```python
from build123d import *

# Parameters (mm, degrees)
SKETCH1_W            = 60
SKETCH1_H            = 7.5
BOSS_EXTRUDE1_DEPTH  = 13
SKETCH3_W            = 12
SKETCH3_H            = 5
CUT_EXTRUDE1_DEPTH   = 10.5
SKETCH4_R            = 1
CUT_EXTRUDE2_DEPTH   = 10
SKETCH9_W            = 45.277568689
SKETCH9_H            = 2.15
CUT_EXTRUDE8_DEPTH   = 15
SKETCH13_W           = 45.277568689
SKETCH13_H           = 3.2
CUT_EXTRUDE10_DEPTH  = 8
SKETCH14_W           = 45.277568689
SKETCH14_H           = 0.95
CUT_EXTRUDE11_DEPTH  = 2.2
RIB10_REACH          = 34.91
SKETCH16_WALL_W      = 80.220727034
SKETCH16_WALL_H      = 1.3
SKETCH20_W           = 12
SKETCH20_H           = 5
BOSS_EXTRUDE3_DEPTH  = 3
SKETCH22_W           = 12
SKETCH22_H           = 5
CUT_EXTRUDE13_DEPTH  = 1.95
CUT_EXTRUDE14_START  = -10
SKETCH23_R           = 1
CUT_EXTRUDE14_DEPTH  = 10
SCALE1_SCALE         = 1.6
SCALE3_SCALE         = 0.8
SCALE4_SCALE         = 0.95890411
SKETCH34_W           = 14.546034326
SKETCH34_H           = 7.999999695
CUT_EXTRUDE20_DEPTH  = 15
SKETCH39_W           = 3.927671232
SKETCH39_H           = 3.436712329
BOSS_EXTRUDE5_DEPTH  = 25
BOSS_EXTRUDE6_DEPTH  = 2
FILLET1_R            = 15
FILLET3_R            = 5
BOSS_EXTRUDE7_DEPTH  = 2
FILLET4_R            = 5
FILLET5_R            = 5
FILLET6_R            = 5
FILLET7_R            = 5
SKETCH52_W           = 9.205479452
SKETCH52_H           = 15.956164384
CUT_EXTRUDE21_DEPTH  = 0.05
SKETCH54_W           = 0.182732797
SKETCH54_H           = 6.136986302
BOSS_EXTRUDE8_DEPTH  = 15
SKETCH55_W           = 6.136986302
SKETCH55_H           = 3.40109589
CUT_EXTRUDE22_DEPTH  = 15
SKETCH57_W           = 14.496034326
SKETCH57_H           = 7.999999695
CUT_EXTRUDE23_DEPTH  = 12.16
SKETCH58_W           = 18.020271855
SKETCH58_H           = 15.956164384
BOSS_EXTRUDE9_DEPTH  = 3
SKETCH59_W           = 18.020271855
SKETCH59_H           = 15.956164384
BOSS_EXTRUDE10_DEPTH = 3


with BuildPart() as part:
    # Sketch1 → Boss-Extrude1 (new body)
    with BuildSketch(Plane(origin=(0, 0, 0), x_dir=(1, 0, 0), z_dir=(0, 1, 0))):
        Rectangle(SKETCH1_W, SKETCH1_H)
    extrude(amount=BOSS_EXTRUDE1_DEPTH)

    # Sketch3 → Cut-Extrude1 (cut)
    with BuildSketch(Plane(origin=(0, 13, 0), x_dir=(1, 0, 0), z_dir=(0, 1, 0))):
        with Locations((-24, 0)):
            Rectangle(SKETCH3_W, SKETCH3_H)
    extrude(amount=-CUT_EXTRUDE1_DEPTH, mode=Mode.SUBTRACT)

    # Sketch4 → Cut-Extrude2 (cut)
    with BuildSketch(Plane(origin=(0, 2.5, 0), x_dir=(1, 0, 0), z_dir=(0, 1, 0))):
        with Locations(Location((-21, 0, 0), (0, 0, 270))):
            Circle(SKETCH4_R)
        with Locations(Location((-26.7, 0, 0), (0, 0, 270))):
            Circle(SKETCH4_R)
    extrude(amount=-CUT_EXTRUDE2_DEPTH, mode=Mode.SUBTRACT)

    # Sketch9 → Cut-Extrude8 (cut)
    with BuildSketch(Plane.XZ):
        with Locations((7.361215656, 2.675)):
            Rectangle(SKETCH9_W, SKETCH9_H)
        with Locations((7.361215656, -2.675)):
            Rectangle(SKETCH9_W, SKETCH9_H)
    extrude(amount=-CUT_EXTRUDE8_DEPTH, mode=Mode.SUBTRACT)

    # Sketch13 → Cut-Extrude10 (cut)
    with BuildSketch(Plane.XZ):
        with Locations((7.361215656, 0)):
            Rectangle(SKETCH13_W, SKETCH13_H)
    extrude(amount=-CUT_EXTRUDE10_DEPTH, mode=Mode.SUBTRACT)

    # Sketch14 → Cut-Extrude11 (cut)
    with BuildSketch(Plane.XZ.offset(-8)):
        with Locations((7.361215656, 1.125)):
            Rectangle(SKETCH14_W, SKETCH14_H)
        with Locations((7.361215656, -1.125)):
            Rectangle(SKETCH14_W, SKETCH14_H)
    extrude(amount=-CUT_EXTRUDE11_DEPTH, mode=Mode.SUBTRACT)

    # Sketch16 wall → Rib10 (add, up to next)
    with BuildSketch(Plane(origin=(-10.539893857, 4, 0), x_dir=(-0.764085816902, -0.645114613389, 0), z_dir=(0.645114613389, -0.764085816902, 0)), mode=Mode.PRIVATE) as rib10_sk1:
        Rectangle(SKETCH16_WALL_W, SKETCH16_WALL_H)
    rib10_tool1 = extrude(rib10_sk1.sketch, amount=-RIB10_REACH, mode=Mode.PRIVATE) - part.part
    add(rib10_tool1.solids().sort_by_distance((-10.539893857, 4, 0))[0])

    # Sketch20 → Boss-Extrude3 (add)
    with BuildSketch(Plane(origin=(0, 2.5, 0), x_dir=(1, 0, 0), z_dir=(0, 1, 0))):
        with Locations((-24, 0)):
            Rectangle(SKETCH20_W, SKETCH20_H)
    extrude(amount=BOSS_EXTRUDE3_DEPTH)

    # Sketch22 → Cut-Extrude13 (cut)
    with BuildSketch(Plane(origin=(0, 5.5, 0), x_dir=(1, 0, 0), z_dir=(0, 1, 0))):
        with Locations((-24, 0)):
            Rectangle(SKETCH22_W, SKETCH22_H)
    extrude(amount=-CUT_EXTRUDE13_DEPTH, mode=Mode.SUBTRACT)

    # Sketch23 → Cut-Extrude14 (cut)
    with BuildSketch(Plane.XZ.offset(CUT_EXTRUDE14_START)):
        with Locations(Location((-26.7, 0, 0), (0, 0, 90))):
            Circle(SKETCH23_R)
        with Locations(Location((-21, 0, 0), (0, 0, 90))):
            Circle(SKETCH23_R)
    extrude(amount=CUT_EXTRUDE14_DEPTH, mode=Mode.SUBTRACT)


with BuildPart() as part_1:
    # Scale1: scaled about (-10.495093685, 7.511594664, 0)
    add(part.part.scale(SCALE1_SCALE).moved(Location((6.297056211, -4.506956798, 0))))


with BuildPart() as part_2:
    # Scale3: scaled about (-10.495093686, 7.511594664, 0)
    add(part_1.part.scale(SCALE3_SCALE).moved(Location((-2.099018737, 1.502318933, 0))))


with BuildPart() as part_3:
    # Scale4: scaled about (-10.495093686, 7.511594664, 0)
    add(part_2.part.scale(SCALE4_SCALE).moved(Location((-0.43130522, 0.308695671, 0))))

    # Sketch34 → Cut-Extrude20 (cut)
    with BuildSketch(Plane(origin=(0, 2.649144227, 0), x_dir=(1, 0, 0), z_dir=(0, 1, 0))):
        with Locations((-27.162345095, -7.59e-07)):
            Rectangle(SKETCH34_W, SKETCH34_H)
    extrude(amount=CUT_EXTRUDE20_DEPTH, mode=Mode.SUBTRACT)

    # Sketch39 → Boss-Extrude5 (add)
    with BuildSketch(Plane(origin=(39.208473359, 0, 0), x_dir=(0, 0, -1), z_dir=(1, 0, 0))):
        with Locations((0, 12.529692173)):
            Rectangle(SKETCH39_W, SKETCH39_H)
    extrude(amount=BOSS_EXTRUDE5_DEPTH)

    # Sketch45 → Boss-Extrude6 (add)
    with BuildSketch(Plane.XY.offset(1.963835616)):
        Polygon((64.208473359, 14.248048337), (67.197905162, 11.258616533), (67.903164447, 7.966965022), (68.244364149, 4.408739558), (65.703189261, 8.649364426), (64.208473359, 10.811336008), align=None)
    extrude(amount=-BOSS_EXTRUDE6_DEPTH)

    # Fillet1
    # the kernel refuses this fillet: 15 mm, written as the material it takes off along each edge
    with BuildSketch(Plane(origin=(67.197905162, 11.258616533, 12.842753048), x_dir=(-0.7071067811865568, 0.7071067811865384, 0), z_dir=(0, 0, -1))) as fillet1_piece_1:
        with BuildLine():
            CenterArc((4.351566973, -15), FILLET1_R, 90, 28.588827617)
            Line((-2.826242727, -1.828855482), (0, 0))
            Line((0, 0), (4.351566973, 0))
        make_face()
    extrude(amount=23.757834864, mode=Mode.SUBTRACT)

    # Fillet3
    fillet3_edges = [part_3.edges().sort_by_distance(p)[0] for p in [
        (64.207755923, 14.248048337, 0),
    ]]
    fillet(fillet3_edges, radius=FILLET3_R)

    # Sketch47 → Boss-Extrude7 (add)
    with BuildSketch(Plane.XY.offset(1.963835616)):
        Polygon((62.681686065, 10.811336008), (65.137458222, 8.07903323), (66.974128155, 4.550150551), (68.244364149, 4.408739558), (65.703189261, 8.649364426), (64.208473359, 10.811336008), align=None)
    extrude(amount=-BOSS_EXTRUDE7_DEPTH)

    # Fillet4
    fillet4_edges = [part_3.edges().sort_by_distance(p)[0] for p in [
        (62.681686065, 10.811336008, 0.963835616),
    ]]
    fillet(fillet4_edges, radius=FILLET4_R)

    # Fillet5
    fillet5_edges = [part_3.edges().sort_by_distance(p)[0] for p in [
        (65.137458222, 8.07903323, 0.963835616),
    ]]
    fillet(fillet5_edges, radius=FILLET5_R)

    # Fillet6
    # the kernel refuses this fillet: 5 mm, written as the material it takes off along each edge
    with BuildSketch(Plane(origin=(68.244364149, 4.408739558, 10.889498263), x_dir=(-0.993860211442073, 0.11064303011178676, 0), z_dir=(0, 0, -1))) as fillet6_piece_1:
        with BuildLine():
            CenterArc((5.625725169, 2.469414691), FILLET6_R, 168.170246518, 41.425870444)
            Line((0.731919855, 3.494436423), (0.634043748, 3.514936858))
            Line((0.634043748, 3.514936858), (-0.097876106, 0.020500435))
            Line((-0.097876106, 0.020500435), (0, -0.1))
            ThreePointArc((0, -0.1), (0.639041577, -0.1), (1.191130314, -0.049388294))
            Line((1.191130314, -0.049388294), (1.278083154, 0))
        make_face()
    extrude(amount=19.851325293, mode=Mode.SUBTRACT)

    # Fillet7
    # the kernel refuses this fillet: 5 mm, written as the material it takes off along each edge
    with BuildSketch(Plane(origin=(39.208473358, 8.111062035, -11.897149471), x_dir=(1.1344900488242768e-10, 1.0, 0), z_dir=(0, 0, 1))) as fillet7_piece_1:
        with BuildLine():
            CenterArc((4.999999999, 4.439736501), FILLET7_R, 180.000000007, 62.61642823)
            Line((-1e-09, 4.439736501), (-0.100000001, 4.439736501))
            Line((-0.100000001, 4.439736501), (-0.1, 0))
            Line((-0.1, 0), (0, -0.1))
            ThreePointArc((0, -0.1), (1.350136986, -0.1), (2.654279452, -0.08879473))
            Line((2.654279452, -0.08879473), (2.700273973, 0))
        make_face()
    extrude(amount=23.794298942, mode=Mode.SUBTRACT)

    # Sketch52 → Cut-Extrude21 (cut)
    with BuildSketch(Plane.ZY.offset(34.435362258)):
        with Locations((0, 6.269966145)):
            Rectangle(SKETCH52_W, SKETCH52_H)
    extrude(amount=-CUT_EXTRUDE21_DEPTH, mode=Mode.SUBTRACT)

    # Sketch54 → Boss-Extrude8 (add)
    with BuildSketch(Plane(origin=(0, 2.649144227, 0), x_dir=(1, 0, 0), z_dir=(0, 1, 0))):
        with Locations((-19.797961534, 0)):
            Rectangle(SKETCH54_W, SKETCH54_H)
    extrude(amount=BOSS_EXTRUDE8_DEPTH)

    # Sketch55 → Cut-Extrude22 (cut)
    with BuildSketch(Plane(origin=(-19.706595135, 0, 0), x_dir=(0, 0, -1), z_dir=(1, 0, 0))):
        with Locations((0, 15.948596282)):
            Rectangle(SKETCH55_W, SKETCH55_H)
    extrude(amount=-CUT_EXTRUDE22_DEPTH, mode=Mode.SUBTRACT)

    # Sketch57 → Cut-Extrude23 (cut)
    with BuildSketch(Plane(origin=(0, 14.248048337, 0), x_dir=(1, 0, 0), z_dir=(0, 1, 0))):
        with Locations((-27.137345095, -7.59e-07)):
            Rectangle(SKETCH57_W, SKETCH57_H)
    extrude(amount=-CUT_EXTRUDE23_DEPTH, mode=Mode.SUBTRACT)

    # Sketch58 → Boss-Extrude9 (add)
    with BuildSketch(Plane.XY.offset(4.602739726)):
        with Locations((-25.37522633, 6.269966145)):
            Rectangle(SKETCH58_W, SKETCH58_H)
    extrude(amount=BOSS_EXTRUDE9_DEPTH)

    # Sketch59 → Boss-Extrude10 (add)
    with BuildSketch(Plane(origin=(0, 0, -4.602739726), x_dir=(-1, 0, 0), z_dir=(0, 0, -1))):
        with Locations((25.37522633, 6.269966145)):
            Rectangle(SKETCH59_W, SKETCH59_H)
    extrude(amount=BOSS_EXTRUDE10_DEPTH)


solid = part_3.part
```
Verification items for the finished model (mm, model axes). A direction names the side the tool comes from. Give positions to 0.01 mm unless a question says otherwise; leave off trailing zeros. Write each loop counter-clockwise with the first axis right and the second up, starting at its lowest first coordinate (ties: lowest second). Pieces come first, ordered by that corner, then holes. Notation, with made-up numbers: (-34, -10) - (-19, -10) arc R37 ccw to (-19, 26) - close; hole circle Ø5 at (39.5, -22). An arc over 180 degrees is marked (long way). Put each result on its own line as item: value.
Q1. Section check D-D on x = -10.5. Record the cut outline in (y, z).
Result:
outline: (3.24, -0.8) - (10.81, -0.8) - (10.81, -1.96) - (14.25, -1.96) - (14.25, 1.96) - (10.81, 1.96) - (10.81, 0.8) - (3.24, 0.8) - close
Q2. Section check A-A on x = 0. Record the cut outline in (y, z), and give its area (3 significant figures).
Result:
outline: (8.11, -0.8) - (10.81, -0.8) - (10.81, -1.96) - (14.25, -1.96) - (14.25, 1.96) - (10.81, 1.96) - (10.81, 0.8) - (8.11, 0.8) - close
area: 17.8 mm2
Q3. Mould release check, pull along Z, two halves, no side actions. Record for faces 6 (the face through (26, 12, 1.964)), 7 (the face through (-31.42, 0.22, 0.66)), 8 (the face through (62.515, 10.366, 0.95)): released by +Z, released by -Z, zero draft, split by the parting line, or undercut.
Result:
face 6: released by +Z
face 7: undercut
face 8: zero draft
Q4. Section check C-C on x = 48.5. Record the cut outline in (y, z).
Result:
outline: (10.81, -1.96) - (14.25, -1.96) - (14.25, 1.96) - (10.81, 1.96) - close
Q5. Scan lines: probe 1 along X at (y, z) = (1.1, 0); probe 2 along X at (y, z) = (-0.8, 0); probe 3 along Z at (x, y) = (-23, 12.75). Record each from-to range of solid material in increasing order. Write a range as from..to.
Result:
probe 1: -34.39..-31.61, -29.16..-24.62, -22.16..-13.04
probe 2: -34.39..-31.61, -29.16..-24.62, -22.16..-15.29
probe 3: -7.6..-4, 4..7.6
Q6. Section check B-B on y = 5.5. Record the cut outline in (x, z).
Result:
outline: (-34.39, -7.6) - (-16.37, -7.6) - (-16.37, -0.8) - (-7.83, -0.8) - (-7.83, 0.8) - (-16.37, 0.8) - (-16.37, 7.6) - (-34.39, 7.6) - (-34.39, 4) - (-19.89, 4) - (-19.89, -4) - (-34.39, -4) - close; (66.48, -0.04) - (67.52, -0.04) - (67.52, 1.96) - (66.48, 1.96) - close
Q7. Set-up check for faces 1 (the face through (-10.47, 3.27, -0.01)), 2 (the face through (23, 10.811, -1)), 3 (the face through (64.208, 12, -1)), 4 (the face through (-27, 2.088, 0)), 5 (the face through (3, 9, 0.798)): record each of +Z, -Z, +X, -X, +Y, -Y from which the full face is reachable in a straight line by a thin tool's end or side.
Result:
face 1: +Z, -Z, -Y
face 2: -Y
face 3: -Z, +X, +Y, -Y
face 4: -X, +Y
face 5: +Z, -Y
Q8. Depth check by flat-ended pin: P1, Ø3, axis at x = 9.5, y = 11.5, coming from the +Z side; P2, Ø0.5, axis at x = 24, z = 0.5, coming from the -Y side; P3, Ø2, axis at y = 9, z = 4.5, coming from the +X side. Enter the tip coordinate at first touch or a pass-through.
Result:
P1: z = 1.96
P2: y = 8.11
P3: x = -16.37
